Job drawing, mm, ordinate dimensions from the low corner. One solid piece. A direction names the side the tool comes from. Round coordinates to 2 decimals unless told otherwise and drop trailing zeros. Loops run counter-clockwise (first coordinate to the right, second up) from the corner with the lowest first, then second, coordinate; pieces in that order, holes last. Notation, with made-up numbers: M 6,-14 L 16,-14 A18 cw 16,-2 Z; hole C 52,66.5 d3. An arc over 180 degrees is marked long. Put each result on its own line as item: value. Start each with the question number.
1) Probe line 1 along Z through (x, y) = (25, 22.8); line 2 along Y through (x, z) = (20.5, 46.5); line 3 along Z through (x, y) = (25, 12.25). List the from-to ranges inside material, lowest first.
2) Slice it at B-B on z = 25. Give the cut face in (x, y).
3) Pull direction X, two halves, no side cores. Call the marked faces 1, 2 and 3: +X half, -X half, draft (parallel to the pull), parting line (faces both ways), or undercut.
4) Slice it at A-A on x = 25. Give the cut face in (y, z).
5) Which spindle directions (+Z, -Z, +X, -X, +Y, -Y) get a long thin tool onto all of the face, cutting with end or side? Do the marked faces 4 and 5. Say none if no direction does.
6) Slice it at D-D on y = 18. Give the cut face in (x, z), then the cut area to 3 significant figures.
7) Drop flat-ended pins along their axis: pin 1 Ø12 at (x, z) = (21, 9) entering from -Y; pin 2 Ø1.5 at (y, z) = (12.5, 25) entering from -X; pin 3 Ø19 at (x, z) = (25, 25) entering from -Y; pin 4 Ø3 at (x, y) = (20.5, 4) entering from +Z. Give the stop position or say it passes through.
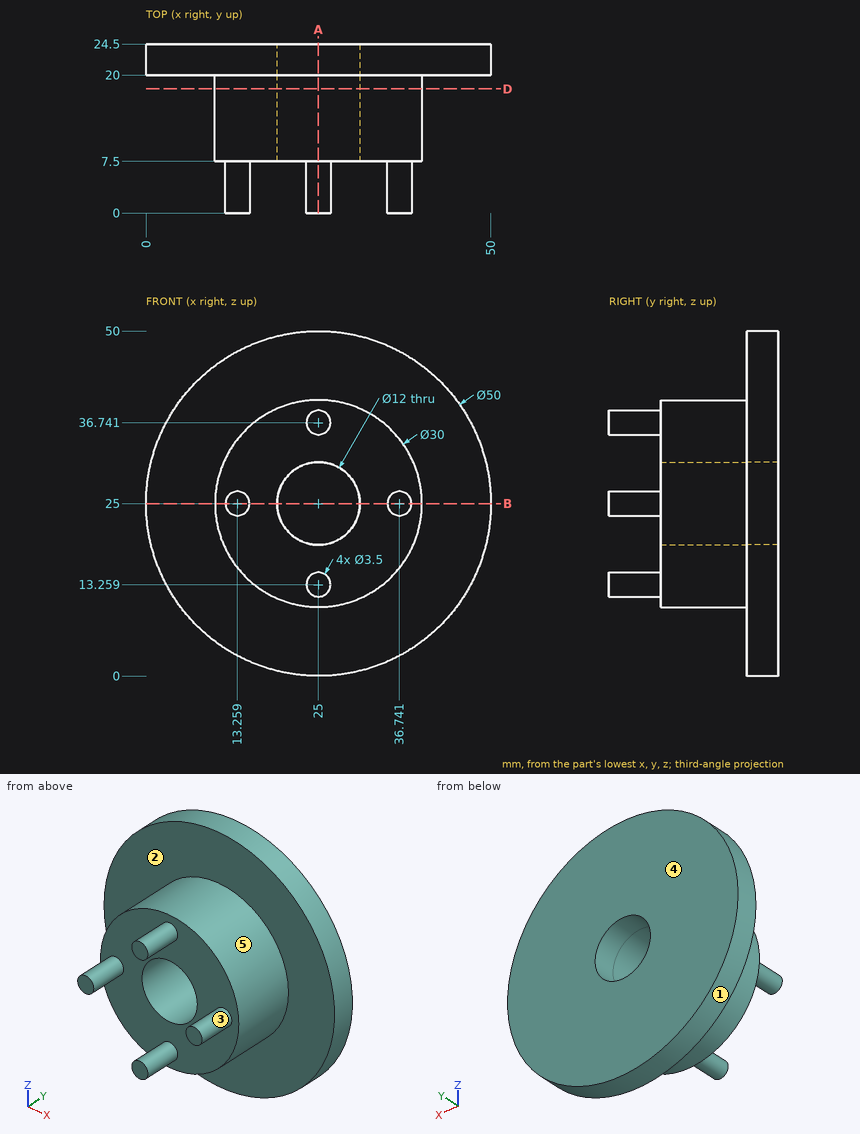
Recorded:
1. line 1: z = 0 to 19, 31 to 50
1. line 2: y = 20 to 24.5
1. line 3: z = 10 to 19, 31 to 40
2. outline: M 0,20 L 10,20 L 10,7.5 L 11.51,7.5 L 11.51,0 L 15.01,0 L 15.01,7.5 L 19,7.5 L 19,24.5 L 0,24.5 Z; M 31,7.5 L 34.99,7.5 L 34.99,0 L 38.49,0 L 38.49,7.5 L 40,7.5 L 40,20 L 50,20 L 50,24.5 L 31,24.5 Z
3. face 1: parting line
3. face 2: draft
3. face 3: undercut
4. outline: M 0,11.51 L 7.5,11.51 L 7.5,10 L 20,10 L 20,0 L 24.5,0 L 24.5,19 L 7.5,19 L 7.5,15.01 L 0,15.01 Z; M 0,34.99 L 7.5,34.99 L 7.5,31 L 24.5,31 L 24.5,50 L 20,50 L 20,40 L 7.5,40 L 7.5,38.49 L 0,38.49 Z
5. face 4: +Z, -Z, +X, -X, +Y
5. face 5: -Y
6. outline: C 25,25 d30; hole C 25,25 d12
6. area: 594 mm2
7. pin 1: stops at y = 0
7. pin 2: stops at x = 10
7. pin 3: stops at y = 7.5
7. pin 4: passes through
